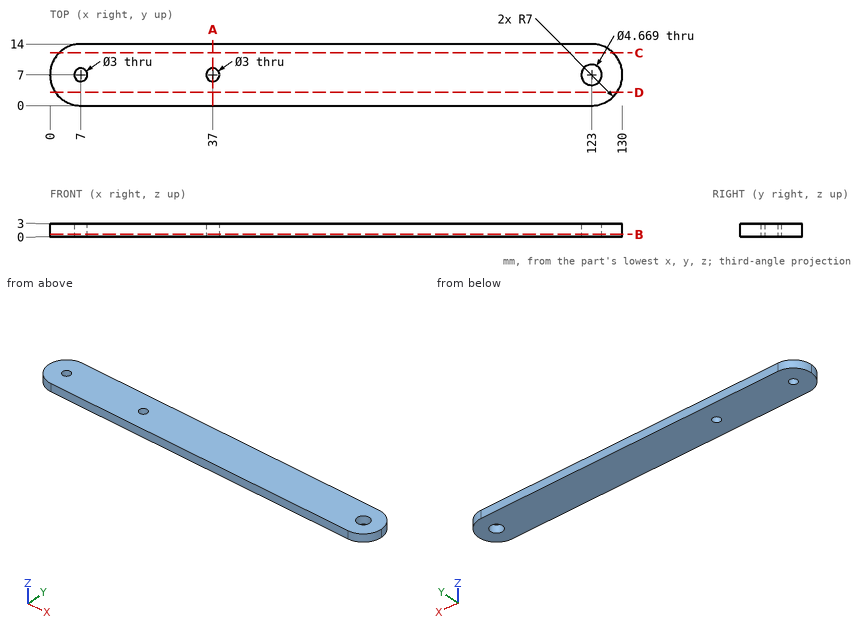
The figure shows three views and two pictorial views of one solid part (mm, origin at its lowest corner). Answer the questions. Give positions to 0.01 mm unless a question says otherwise; leave off trailing zeros. Order: outer loops, then holes, each group sorted by start corner. A loop starts at its lowest first (then second) coordinate and runs counter-clockwise, first axis right, second up. Notation, with made-up numbers: (-16, 44) -> (37, 44) arc R38 cw to (37, 83) -> close; hole circle Ø5 at (53.25, -27.75). An arc over 180 degrees is marked (long way). Answer as a JSON object with one key per item and string values. Group by question number.
Item 1: The part is cut by section D-D on y = 3. Write down the section's boundary in (x, z).
Item 2: Consider L1, parallel to Y at x = 123, z = 0.9; L2, parallel to Y at x = 7, z = 0.9; L3, parallel to X at y = 11, z = 0.8 (1 decimal). Determine where each line is inside the solid, lowest interval first. Write a range as from..to.
Item 3: The part is cut by section B-B on z = 0.55. Write down the section's boundary in (x, y), and give its area (3 significant figures).
Item 4: The part is cut by section C-C on y = 12. Write down the section's boundary in (x, z).
Item 5: A flat-ended cylindrical pin translates along its axis: pin 1 (4 mm diameter, centred on x = 123, y = 7, fed in from +Z). Find the tip coordinate at first contact, or state that the pin passes through.
Item 6: The part is cut by section A-A on x = 37. Write down the section's boundary in (y, z), and give its area (3 significant figures).
Result set:
{
 "1": {"outline": "(1.26, 0) -> (128.74, 0) -> (128.74, 3) -> (1.26, 3) -> close"},
 "2": {"L1": "0..4.67, 9.33..14", "L2": "0..5.5, 8.5..14", "L3": "1.3..128.7"},
 "3": {"outline": "(0, 7) arc R7 ccw to (7, 0) -> (123, 0) arc R7 ccw to (130, 7) arc R7 ccw to (123, 14) -> (7, 14) arc R7 ccw to start; hole circle Ø3 at (7, 7); hole circle Ø3 at (37, 7); hole circle Ø4.67 at (123, 7)", "area": "1,750 mm²"},
 "4": {"outline": "(2.1, 0) -> (127.9, 0) -> (127.9, 3) -> (2.1, 3) -> close"},
 "5": {"pin 1": "through"},
 "6": {"outline": "(0, 0) -> (5.5, 0) -> (5.5, 3) -> (0, 3) -> close; (8.5, 0) -> (14, 0) -> (14, 3) -> (8.5, 3) -> close", "area": "33.0 mm²"}
}
